Source: three-view drawing plus pictorial views. Frame: mm from the lowest corner of the part. A direction names the side the tool comes from. Give positions to 0.01 mm unless a question says otherwise; leave off trailing zeros. Loops run counter-clockwise (first coordinate to the right, second up) from the corner with the lowest first, then second, coordinate; pieces in that order, holes last. Notation, with made-up numbers: (51, 62.5) - (70, 62.5) arc R25 cw to (70, 97.5) - close; hole circle Ø7 at (-18.75, 9.5). An arc over 180 degrees is marked (long way). Answer as a JSON object with one key per item and string values.
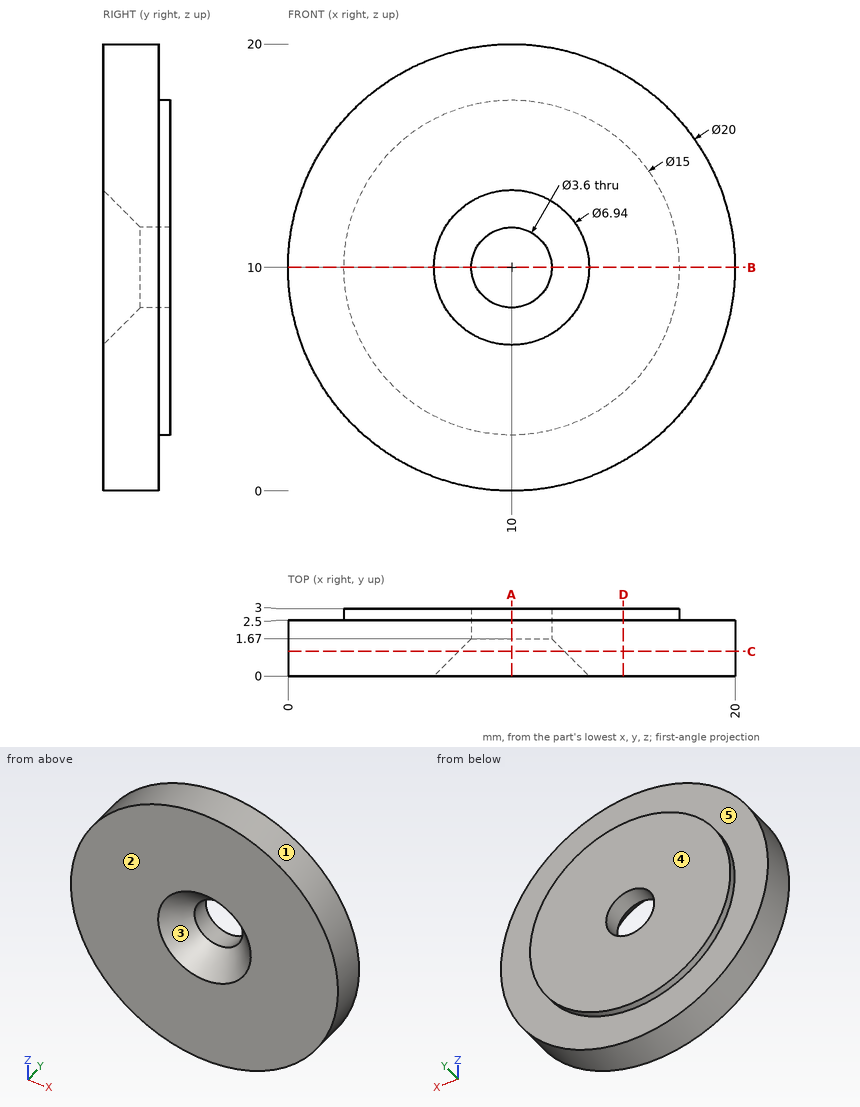
Item 1: Contact query for flat-ended pins moving along their axis: P1, Ø1.5, axis at y = 2.5, z = 12.5, coming from the +X side; P2, Ø1.5, axis at y = 2, z = 7, coming from the -X side. Output: stop coordinate, or through.
Geometry check:
{"P1": "stops at x = 19.85", "P2": "stops at x = 0.26"}
Item 2: Cut plane B-B (z = 10). Return loops of the section in (x, y), then the cut area to 3 significant figures.
Geometry check:
{"outline": "(0, 0) - (6.53, 0) - (8.2, 1.67) - (8.2, 3) - (2.5, 3) - (2.5, 2.5) - (0, 2.5) - close; (11.8, 1.67) - (13.47, 0) - (20, 0) - (20, 2.5) - (17.5, 2.5) - (17.5, 3) - (11.8, 3) - close", "area": "43.9 mm2"}
Item 3: Cut plane A-A (x = 10). Return loops of the section in (y, z).
Geometry check:
{"outline": "(0, 0) - (2.5, 0) - (2.5, 2.5) - (3, 2.5) - (3, 8.2) - (1.67, 8.2) - (0, 6.53) - close; (0, 13.47) - (1.67, 11.8) - (3, 11.8) - (3, 17.5) - (2.5, 17.5) - (2.5, 20) - (0, 20) - close"}
Item 4: Access query for the marked faces 4 and 5. Directions: +Z, -Z, +X, -X, +Y, -Y. A direction counts if a zero-diameter tool reaches every point of the face in a straight line with its end or side. Return the directions, or none.
Geometry check:
{"face 4": "+Z, -Z, +X, -X, +Y", "face 5": "+Y"}
Item 5: Material intervals for line 1 (X direction, y = 2.15, z = 10); line 2 (X direction, y = 2.7, z = 10); line 3 (Y direction, x = 17.5, z = 12.5), sorted ascending. Write a range as [from, to].
Geometry check:
{"line 1": "x = [0, 8.2], [11.8, 20]", "line 2": "x = [2.5, 8.2], [11.8, 17.5]", "line 3": "y = [0, 2.5]"}
Item 6: Cut plane C-C (y = 1.1). Return loops of the section in (x, z).
Geometry check:
{"outline": "circle Ø20 at (10, 10); hole circle Ø4.74 at (10, 10)"}
Item 7: Cut plane D-D (x = 15). Return loops of the section in (y, z), then the cut area to 3 significant figures.
Geometry check:
{"outline": "(0, 1.34) - (2.5, 1.34) - (2.5, 4.41) - (3, 4.41) - (3, 15.59) - (2.5, 15.59) - (2.5, 18.66) - (0, 18.66) - close", "area": "48.9 mm2"}
Item 8: Mould query, pull axis X, two halves, no side actions, for the marked faces 1, 2 and 3. Classes: released by +X, released by -X, zero draft, split by the parting line, or undercut.
Geometry check:
{"face 1": "split by the parting line", "face 2": "zero draft", "face 3": "undercut"}
